```python
from build123d import *

# Parameters (mm, degrees)
F0_R     = 76.2
F1_DEPTH = 19.05


# Not quite as in the source:
# - a length typed as a fraction of an inch, garbled in the dataset ("3 / 203.2 mm" for 3/8 in), is restored
# - a feature names something its author has since deleted; it is built from what else it names


with BuildPart() as f1:
    # F0 (on Front) → F1 (new body)
    with BuildSketch(Plane.XZ):
        Polygon((-277.4270822048, 25.2823245883), (-277.4270822048, -76.3176754117), (-175.8270822048, -76.3176754117), (-125.0270822048, -26.4387615025), (-23.4270822048, -26.4387615025), (27.3729177952, -76.3176754117), (128.9729177952, -76.3176754117), (126.3909138083, 26.5286043286), (100.9909138083, 26.5286043286), (100.9909138083, 128.1286043286), (126.3909138083, 128.1286043286), (126.3909138083, 584.0823245883), (103.5729177952, 584.0823245883), (103.5729177952, 685.6823245883), (128.9729177952, 685.6823245883), (128.9729177952, 787.2823245883), (21.0229177952, 787.2823245883), (21.0229177952, 761.8823245883), (-169.4770822048, 761.8823245883), (-169.4770822048, 787.2823245883), (-277.4270822048, 787.2823245883), (-277.4270822048, 685.6823245883), (-252.0270822048, 685.6823245883), (-252.0270822048, 584.0823245883), (-277.4270822048, 584.0823245883), (-277.4270822048, 126.8823245883), (-252.0270822048, 126.8823245883), (-252.0270822048, 25.2823245883), align=None)
        with Locations((-52.0020822048, 355.4823245883)):
            Circle(F0_R, mode=Mode.SUBTRACT)
    extrude(amount=F1_DEPTH)


solid = f1.part
```
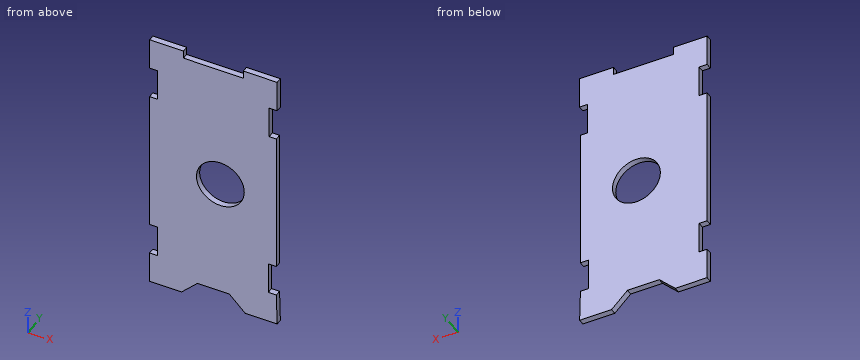
Input: part model. Units: mm. Frame: model coordinates. Round coordinates to 2 decimals unless told otherwise and drop trailing zeros. Order: outer loops, then holes, each group sorted by start corner. A loop starts at its lowest first (then second) coordinate and runs counter-clockwise, first axis right, second up. Notation, with made-up numbers: (83, 34.25) - (108, 34.25) arc R27 cw to (108, 71.25) - close; hole circle Ø10 at (-14, 62). An arc over 180 degrees is marked (long way). Answer in a Markdown table with one row per item.
Item 1: Section query A-A (x = -45). Return the cut outline in (y, z), then the cut area to 3 significant figures.
Model answer:
| item | result |
|---|---|
| outline | (-19.05, -26.44) - (0, -26.44) - (0, 279.6) - (-19.05, 279.6) - close; (-19.05, 431.36) - (0, 431.36) - (0, 761.88) - (-19.05, 761.88) - close |
| area | 12,100 mm² |
Item 2: Line query: line 1 (X direction, y = -11.5, z = 573.5); line 2 (Z direction, x = -26, y = -8.75); line 3 (X direction, y = -13.5, z = 374). Output: solid intervals per line, ascending.
Model answer:
| item | result |
|---|---|
| line 1 | x = -277.43 to 126.39 |
| line 2 | z = -26.44 to 283.86, 427.11 to 761.88 |
| line 3 | x = -277.43 to -125.92, 21.91 to 126.39 |
Item 3: Section query D-D (z = 102). Return the cut outline in (x, y), then the cut area to 4 significant figures.
Model answer:
| item | result |
|---|---|
| outline | (-252.03, -19.05) - (100.99, -19.05) - (100.99, 0) - (-252.03, 0) - close |
| area | 6,725 mm² |
Item 4: Pin query (flat end, axial travel): pin 1 (5.5 mm diameter, centred on y = -11.5, z = 617, fed in from +X); pin 2 (3 mm diameter, centred on x = -34.5, y = -7, fed in from +Z); pin 3 (3 mm diameter, centred on y = -4, z = 467, fed in from +X). Return the tip coordinate at first contact, or that it passes through.
Model answer:
| item | result |
|---|---|
| pin 1 | stops at x = 103.57 |
| pin 2 | stops at z = 761.88 |
| pin 3 | stops at x = 126.39 |
Item 5: Section query B-B (z = 368). Return the cut outline in (x, y).
Model answer:
| item | result |
|---|---|
| outline | (-277.43, -19.05) - (-127.17, -19.05) - (-127.17, 0) - (-277.43, 0) - close; (23.16, -19.05) - (126.39, -19.05) - (126.39, 0) - (23.16, 0) - close |
